Design review of the part shown in the three views and the two pictorial views. Dimensions are in mm from the part's minimum x, y and z. Round coordinates to 2 decimals unless told otherwise and drop trailing zeros. Order: outer loops, then holes, each group sorted by start corner. A loop starts at its lowest first (then second) coordinate and runs counter-clockwise, first axis right, second up. Notation, with made-up numbers: M -37.5,50 L -13.5,50 A36 cw -13.5,89 Z; hole C 73,-35.5 d10. An arc over 180 degrees is marked long. Use a Markdown table: item, result. Add a question column.
(1) Take a section at C-C (x = 54). Write out the cut boundary in (y, z).
(2) For pin 1 (3 mm diameter, centred on x = 22, y = 29.5, fed in from +Z); pin 2 (1 mm diameter, centred on x = 36, z = 8.5, fed in from -Y), all flat-tipped, find the tip position at first contact; note any pin that passes through.
(3) Take a section at B-B (y = 71.1). Write out the cut boundary in (x, z) (3 decimals).
(4) To check wall thickness, follow probe 1 along Z at (x, y) = (23, 44.5); probe 2 along X at (y, z) = (7, 3) (3 decimals); probe 3 along Y at (x, z) = (63, 6.25). State the ranges of each line that lie inside material, in increasing order. Write a range as from..to.
(5) Take a section at D-D (z = 21.5). Write out the cut boundary in (x, y) (3 decimals), then the cut area to 3 significant figures.
(6) Take a section at A-A (z = 7.75). Write out the cut boundary in (x, y) (3 decimals), then the cut area to 3 significant figures.
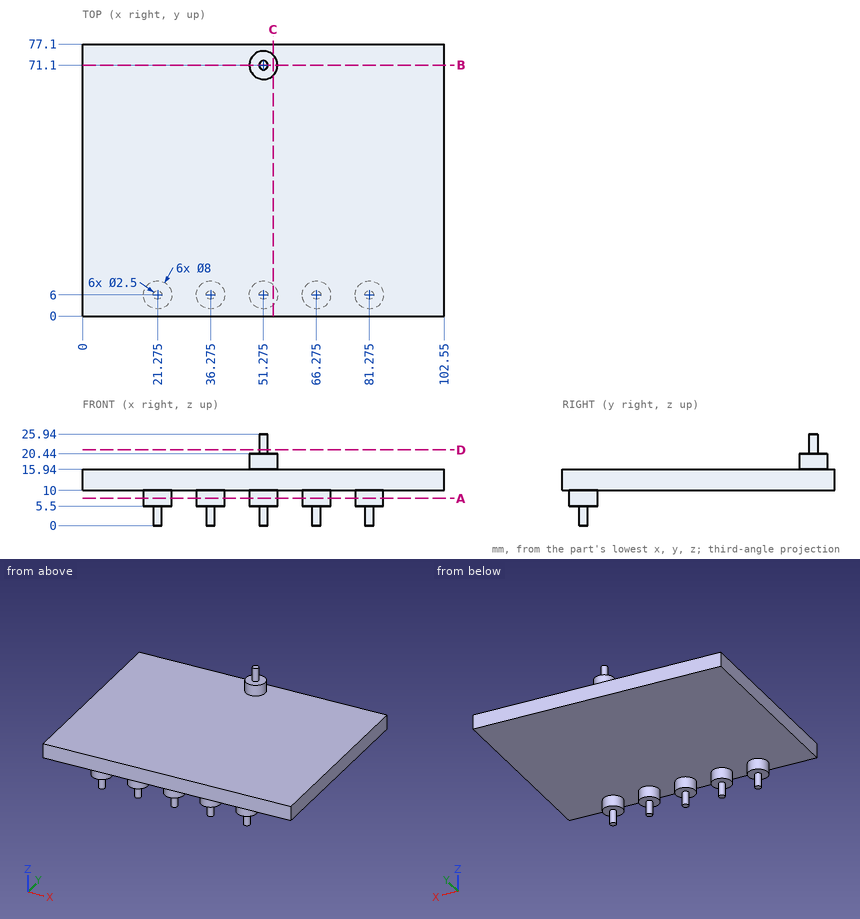
Verdict:
| question | item | result |
|---|---|---|
| 1 | outline | M 0,10 L 3.07,10 L 3.07,5.5 L 8.93,5.5 L 8.93,10 L 77.1,10 L 77.1,15.94 L 74.03,15.94 L 74.03,20.44 L 68.17,20.44 L 68.17,15.94 L 0,15.94 Z |
| 2 | pin 1 | stops at z = 15.94 |
| 2 | pin 2 | stops at y = 2 |
| 3 | outline | M 0,10 L 102.55,10 L 102.55,15.94 L 55.275,15.94 L 55.275,20.44 L 52.525,20.44 L 52.525,25.94 L 50.025,25.94 L 50.025,20.44 L 47.275,20.44 L 47.275,15.94 L 0,15.94 Z |
| 4 | probe 1 | z = 10..15.94 |
| 4 | probe 2 | x = 20.525..22.025, 35.525..37.025, 50.525..52.025, 65.525..67.025, 80.525..82.025 |
| 4 | probe 3 | y = 3.7..8.3 |
| 5 | outline | C 51.275,71.1 d2.5 |
| 5 | area | 4.91 mm^2 |
| 6 | outline | C 21.275,6 d8; C 36.275,6 d8; C 51.275,6 d8; C 66.275,6 d8; C 81.275,6 d8 |
| 6 | area | 251 mm^2 |
